from build123d import *

# Parameters (mm, degrees)
ESBO_O1_R                = 2.95
RESSALTO_EXTRUS_O1_DEPTH = 17.6
RESSALTO_EXTRUS_O2_START = -20.5
RESSALTO_EXTRUS_O2_DEPTH = 20.5
FILETE1_R                = 1.5
ESBO_O3_R                = 3.25
CORTE_EXTRUS_O1_DEPTH    = 22.699009104
ESBO_O5_R                = 3.25
ESBO_O5_R_2              = 2.1
RESSALTO_EXTRUS_O3_DEPTH = 9.1
CHANFRO1_SIZE            = 1.2


with BuildPart() as part:
    # Esboço1 → Ressalto-extrusão1 (new, symmetric)
    with BuildSketch(Plane(origin=(0, 0, 0), x_dir=(0, 0, -1), z_dir=(1, 0, 0))):
        with BuildLine():
            Line((5.15, -6.450193796), (-5.15, -6.450193796))
            Line((-5.15, -6.450193796), (-5.15, 0))
            ThreePointArc((-5.15, 0), (0, 5.15), (5.15, 0))
            Line((5.15, 0), (5.15, -6.450193796))
        make_face()
        Circle(ESBO_O1_R, mode=Mode.SUBTRACT)
    extrude(amount=RESSALTO_EXTRUS_O1_DEPTH, both=True)

    # Esboço2 → Ressalto-extrusão2 (add)
    with BuildSketch(Plane.ZY.offset(17.6).offset(RESSALTO_EXTRUS_O2_START)):
        with BuildLine():
            Line((-5.15, 0), (-5.15, -6.450193796))
            Line((-5.15, -6.450193796), (5.15, -6.450193796))
            Line((5.15, -6.450193796), (5.15, 0))
            ThreePointArc((5.15, 0), (0, 5.15), (-5.15, 0))
        make_face()
    extrude(amount=RESSALTO_EXTRUS_O2_DEPTH)

    # Filete1
    filete1_edges = [part.edges().sort_by_distance(p)[0] for p in [
        (-17.6, -3.225096898, -5.15),
        (-17.6, -3.225096898, 5.15),
        (-17.6, 5.15, 0),
    ]]
    fillet(filete1_edges, radius=FILETE1_R)

    # Esboço3 → Corte-extrusão1 (cut, through all)
    with BuildSketch(Plane.XZ.offset(6.450193796)):
        with Locations(Location((-11.3, 0, 0), (0, 0, 270))):
            Circle(ESBO_O3_R)
        with Locations(Location((-0.8, 0, 0), (0, 0, 270))):
            Circle(ESBO_O3_R)
    extrude(amount=-CORTE_EXTRUS_O1_DEPTH, mode=Mode.SUBTRACT)

    # Esboço5 → Ressalto-extrusão3 (add)
    # profile 1 of 2: a face of its own
    with BuildSketch(Plane.XZ.offset(6.450193796)):
        with Locations(Location((-0.8, 0, 0), (0, 0, 270))):
            Circle(ESBO_O5_R)
        with Locations(Location((-0.8, 0, 0), (0, 0, 270))):
            Circle(ESBO_O5_R_2, mode=Mode.SUBTRACT)
    # profile 2 of 2: a face of its own
    with BuildSketch(Plane.XZ.offset(6.450193796)):
        with Locations(Location((-11.3, 0, 0), (0, 0, 270))):
            Circle(ESBO_O5_R)
        with Locations(Location((-11.3, 0, 0), (0, 0, 270))):
            Circle(ESBO_O5_R_2, mode=Mode.SUBTRACT)
    extrude(amount=-RESSALTO_EXTRUS_O3_DEPTH)

    # Chanfro1
    # the kernel refuses this chamfer: 1.2 mm, written as the material it takes off along each edge
    with BuildSketch(Plane(origin=(-11.3, 2.649806204, 0), x_dir=(0, 0, -1), z_dir=(-1, 0, 0))) as chanfro1_piece_1_section:
        Polygon((2.1 + CHANFRO1_SIZE, 0), (2.1, CHANFRO1_SIZE), (2.1, 0), align=None)
    chanfro1_piece_1 = revolve(axis=Axis((-11.3, 2.649806204, 0), (0, -1, 0)), mode=Mode.PRIVATE)
    chanfro1_piece_1 = chanfro1_piece_1 & Plane(origin=(-11.3, 2.024165302, 0), x_dir=(0, 0, -1), z_dir=(0, -1, 0)) * Cylinder(3.25, 14, mode=Mode.PRIVATE)
    add(chanfro1_piece_1, mode=Mode.SUBTRACT)
    with BuildSketch(Plane(origin=(-0.8, 2.649806204, 0), x_dir=(0, 0, -1), z_dir=(-1, 0, 0))) as chanfro1_piece_2_section:
        Polygon((2.1 + CHANFRO1_SIZE, 0), (2.1, CHANFRO1_SIZE), (2.1, 0), align=None)
    chanfro1_piece_2 = revolve(axis=Axis((-0.8, 2.649806204, 0), (0, -1, 0)), mode=Mode.PRIVATE)
    chanfro1_piece_2 = chanfro1_piece_2 & Plane(origin=(-0.8, 2.024165302, 0), x_dir=(0, 0, -1), z_dir=(0, -1, 0)) * Cylinder(3.25, 14, mode=Mode.PRIVATE)
    add(chanfro1_piece_2, mode=Mode.SUBTRACT)


solid = part.part
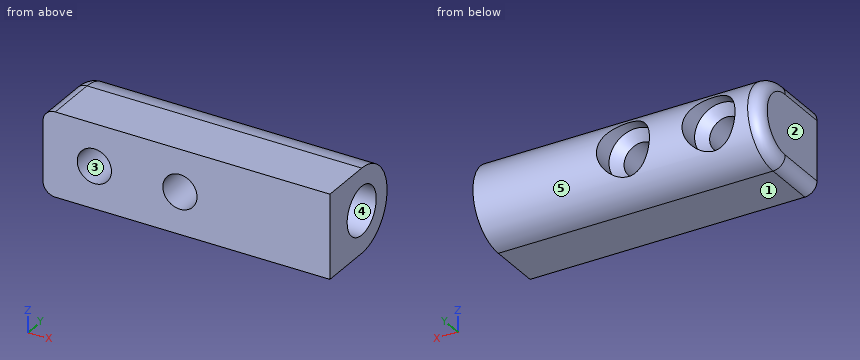
The model under review builds one solid part; all positions refer to its coordinate system, in mm. Face numbers are marked on the shaded views. A direction names the side the tool comes from. Round coordinates to 2 decimals unless told otherwise and drop trailing zeros. Write each loop counter-clockwise with the first axis right and the second up, starting at its lowest first coordinate (ties: lowest second). Pieces come first, ordered by that corner, then holes. Notation, with made-up numbers: M 67,60.5 L 96,60.5 A9 cw 96,67.5 Z; hole C -39.5,44.25 d4. An arc over 180 degrees is marked long. Answer as CSV lines item,"result". Start each with the question number.
Q1. Tool access review of the marked faces 4 and 5: name each direction out of +Z, -Z, +X, -X, +Y, -Y from which nothing blocks a thin tool from reaching the whole face with its end or side.
Q2. Consider section C-C, the plane x = -11.3. Give the boundary of the cut face in (y, z) (3 decimals), then the cut area to 3 significant figures.
Q3. Consider section D-D, the plane x = -7. Give the boundary of the cut face in (y, z).
Q4. Clearance check with flat-ended pins moving along their axes: P1, Ø3.5, axis at x = -11.3, z = 0, coming from the +Y side; P2, Ø3, axis at x = -11.5, z = 4, coming from the +Y side; P3, Ø1.8, axis at y = 0, z = 0.5, coming from the +X side. State where each tip first meets the part, or that it passes through.
Q5. Consider section A-A, the plane z = 0. Give the boundary of the cut face in (x, y).
Q6. The part is to be moulded in two halves that separate along X. For the marked faces 1, 2 and 3, say which applies: +X half, -X half, draft (parallel to the pull), parting line (faces both ways), or undercut.
Q7. Consider section B-B, the plane x = 13. Give the boundary of the cut face in (y, z), then the cut area to 3 significant figures.
Q8. Wall thickness on line 1 along X through (y, z) = (-4.5, 0); line 2 along X through (y, z) = (3.6, 0); line 3 along Z through (x, y) = (3, 0): over which ranges is each line inside the solid? List them lowest first.
Result set:
1,face 4,"+X"
1,face 5,"+X, -X, +Y"
2,outline,"M -6.45,-5.15 L 0,-5.15 A5.15 ccw 3.995,-3.25 L 2.6,-3.25 L 1.45,-2.1 L -6.45,-2.1 Z; M -6.45,2.1 L 1.45,2.1 L 2.6,3.25 L 3.995,3.25 A5.15 ccw 0,5.15 L -6.45,5.15 Z"
2,area,"54.6 mm²"
3,outline,"M -6.45,-5.15 L 0,-5.15 A5.15 ccw 0,5.15 L -6.45,5.15 Z"
4,P1,"passes through"
4,P2,"stops at y = 4.2"
4,P3,"stops at x = 2.9"
5,outline,"M -17.6,-6.45 L -13.4,-6.45 L -13.4,1.45 L -14.55,2.6 L -14.55,5.15 L -16.1,5.15 A1.5 ccw -17.6,3.65 Z; M -9.2,-6.45 L -2.9,-6.45 L -2.9,1.45 L -4.05,2.6 L -4.05,5.15 L -8.05,5.15 L -8.05,2.6 L -9.2,1.45 Z; M 1.3,-6.45 L 17.6,-6.45 L 17.6,-2.95 L 2.9,-2.95 L 2.9,2.95 L 17.6,2.95 L 17.6,5.15 L 2.45,5.15 L 2.45,2.6 L 1.3,1.45 Z"
6,face 1,"draft"
6,face 2,"-X half"
6,face 3,"undercut"
7,outline,"M -6.45,-5.15 L 0,-5.15 A5.15 ccw 0,5.15 L -6.45,5.15 Z; hole C 0,0 d5.9"
7,area,"80.8 mm²"
8,line 1,"x = -17.6 to -13.4, -9.2 to -2.9, 1.3 to 17.6"
8,line 2,"x = -17.6 to -14.55, -8.05 to -4.05, 2.45 to 17.6"
8,line 3,"z = -5.15 to -2.95, 2.95 to 5.15"
